The listing builds one solid part. Answer for the finished solid, in the listing's coordinates (mm). A direction names the side the tool comes from. Give positions to 0.01 mm unless a question says otherwise; leave off trailing zeros. Loops run counter-clockwise (first coordinate to the right, second up) from the corner with the lowest first, then second, coordinate; pieces in that order, holes last. Notation, with made-up numbers: (61.25, -36) - (78.25, -36) arc R30 cw to (78.25, -9) - close; hole circle Ø9 at (89, 29). An arc over 180 degrees is marked (long way). Write item = value, one per line. Start each with the question number.
1) The part is cut by section C-C on x = -7.25. Write down the section's boundary in (y, z), plus the area to 3 significant figures.
2) The part is cut by section B-B on y = -8. Write down the section's boundary in (x, z).
3) The part is cut by section A-A on z = -1.5. Write down the section's boundary in (x, y).
4) The part is cut by section D-D on z = 14.5. Write down the section's boundary in (x, y).
5) Consider probe 1 along Y at (x, z) = (0, 1.25); probe 2 along X at (y, z) = (8, -3.65). Determine where each line is inside the solid, lowest interval first.
6) Flat-ended cylindrical pins translate along their axes: P1, Ø8, axis at x = -3, z = -1.5, coming from the -Y side; P2, Ø3, axis at x = -4, z = 5.5, coming from the -Y side; P3, Ø1.5, axis at x = -0.5, y = 1.5, coming from the -Z side. Find the tip coordinate at first contact, or state that the pin passes through.
7) The mould has two halves that part along X. Classify faces 1 (the cylindrical face through (9.216, -9.115, -2.958)), 2 (the cylindrical face through (-6.69, 9, -2.96)), 3 (the cylindrical face through (6.691, -12.864, -2.958)), 4 (the flat face through (0, 0, 28)): +X half, -X half, draft (parallel to the pull), parting line (faces both ways), or undercut.
8) Which of the six approach directions +Z, -Z, +X, -X, +Y, -Y give full straight-line access (tool end or side, diameter ignored) to faces 5 (the cylindrical face through (0.75, -5.7, 7.18)), 6 (the cylindrical face through (9.65, 7.93, -2.96)), 7 (the cylindrical face through (5.96, 1.88, 13.8))?
from build123d import *

# Parameters (mm, degrees)
F0_R     = 14.5
F0_R_2   = 6.25
F1_DEPTH = 6
F2_DEPTH = 28
F4_D     = 3.3
F5_D     = 11.5
F5_DEPTH = 26
F5_TIP   = 3.4549485594


with BuildPart() as f1:
    # F0 (on Top) → F1 (new body)
    with BuildSketch(Plane.XY):
        Circle(F0_R)
        Circle(F0_R_2, mode=Mode.SUBTRACT)
        Circle(F0_R_2)
    extrude(amount=-F1_DEPTH)

    # F0 (on Top) → F2 (join)
    with BuildSketch(Plane.XY):
        Circle(F0_R_2)
    extrude(amount=F2_DEPTH)

    # F4 (through all)
    with Locations(Plane(origin=(0, 0, -6), x_dir=(1, 0, 0), z_dir=(0, 0, -1))):
        with Locations((8, 8), (8, -8), (-8, -8), (-8, 8)):
            Hole(F4_D / 2)

    # F5
    with Locations(Plane(origin=(0, 0, -6), x_dir=(1, 0, 0), z_dir=(0, 0, -1))):
        with Locations((0, 0)):
            Hole(F5_D / 2, depth=F5_DEPTH)
            with Locations((0, 0, -(F5_DEPTH + F5_TIP / 2))):  # 118° drill point
                Cone(0, F5_D / 2, F5_TIP, mode=Mode.SUBTRACT)


solid = f1.part
Answer below:
q1.outline = (-12.56, -6) - (-9.47, -6) - (-9.47, 0) - (-12.56, 0) - close; (-6.53, -6) - (6.53, -6) - (6.53, 0) - (-6.53, 0) - close; (9.47, -6) - (12.56, -6) - (12.56, 0) - (9.47, 0) - close
q1.area = 115 mm2
q2.outline = (-12.09, -6) - (-9.65, -6) - (-9.65, 0) - (-12.09, 0) - close; (-6.35, -6) - (6.35, -6) - (6.35, 0) - (-6.35, 0) - close; (9.65, -6) - (12.09, -6) - (12.09, 0) - (9.65, 0) - close
q3.outline = circle Ø29 at (0, 0); hole circle Ø3.3 at (-8, -8); hole circle Ø3.3 at (-8, 8); hole circle Ø11.5 at (0, 0); hole circle Ø3.3 at (8, -8); hole circle Ø3.3 at (8, 8)
q4.outline = circle Ø12.5 at (0, 0); hole circle Ø11.5 at (0, 0)
q5.probe_1 = -6.25 to -5.75, 5.75 to 6.25
q5.probe_2 = -12.09 to -9.65, -6.35 to 6.35, 9.65 to 12.09
q6.P1 = -14.5
q6.P2 = -5.73
q6.P3 = 22.05
q7.face_1 = undercut
q7.face_2 = undercut
q7.face_3 = parting line
q7.face_4 = draft
q8.face_5 = -Z
q8.face_6 = +Z, -Z
q8.face_7 = +Z
